Autodesk Inventor part; units mm, degrees
ref_plane "YZ Plane" through (0, 0, 0) normal (1, 0, 0) x (0, 1, 0)
ref_plane "XZ Plane" through (0, 0, 0) normal (0, 1, 0) x (-1, 0, 0)
ref_plane "XY Plane" through (0, 0, 0) normal (0, 0, 1) x (1, 0, 0)
sketch "Эскиз1" plane through (0, 0, 0) normal (0, 0, 1) x (1, 0, 0)
  circle A0 centre (0, 0) radius 40
  line L0 (-40, 0) -> (-13.6038, 219.402)
  line L1 (-13.6038, 219.402) -> (13.6038, 219.402)
  line L2 (13.6038, 219.402) -> (40, 0)
  line L3 (0, 0) -> (0, 40) construction
  line L4 (0, 0) -> (40, 0) construction
  point P0 (0, 219.402)
  dimension "d0" = 80
extrude "Выдавливание1" add sketch "Эскиз1" along normal blind 3 contours L0 A0 L2 | L0 L1 L2 A0
sketch "Эскиз2" plane through (0, 0, 3) normal (0, 0, 1) x (1, 0, 0)
  arc A0 (3, 2.25) -> (-3, 2.25) centre (0, 0) ccw construction
  line L0 (-1.9929, 14.1684) -> (-3, 2.25) construction
  arc A1 (1.9929, 14.1684) -> (-1.9929, 14.1684) centre (0, 14) ccw construction
  line L1 (3, 2.25) -> (1.9929, 14.1684) construction
  circle A2 centre (0, 13) radius 0.5 construction
  circle A3 centre (0, 11) radius 0.5 construction
  circle A4 centre (0, 9) radius 0.5 construction
  circle A5 centre (0, 7) radius 0.5 construction
  circle A6 centre (0, 5) radius 0.5 construction
  circle A7 centre (0, 15) radius 0.5 construction
  arc A8 (-1.9929, -14.1684) -> (1.9929, -14.1684) centre (0, -14) ccw construction
  line L2 (-3, -2.25) -> (-1.9929, -14.1684) construction
  arc A9 (-3, -2.25) -> (3, -2.25) centre (0, 0) ccw construction
  line L3 (1.9929, -14.1684) -> (3, -2.25) construction
  circle A10 centre (0, -5) radius 0.5 construction
  circle A11 centre (0, -7) radius 0.5 construction
  circle A12 centre (0, -9) radius 0.5 construction
  circle A13 centre (0, -11) radius 0.5 construction
  circle A14 centre (0, -13) radius 0.5 construction
  circle A15 centre (0, -15) radius 0.5 construction
  circle A16 centre (0, 0) radius 2.3
  circle A17 centre (0, 9) radius 1
  circle A18 centre (0, -9) radius 1
  point P0 (0, 0)
  dimension "d3" = 2
  dimension "d4" = 2
extrude "Выдавливание2" cut sketch "Эскиз2" against normal blind 10
properties part number "ухо"
Check sheet for the modelled part. Datum: model origin and axes. Units: mm. Give positions to 0.01 mm unless a question says otherwise; leave off trailing zeros. Order: outer loops, then holes, each group sorted by start corner. A loop starts at its lowest first (then second) coordinate and runs counter-clockwise, first axis right, second up. Notation, with made-up numbers: M 56,32 L 97,32 A22 cw 97,40 Z; hole C -9.75,17.5 d11. An arc over 180 degrees is marked long. Answer in a Markdown table with one row per item.
1) Cross-section at A-A, the plane z = 0.8. Enter the section's corners in (x, y).
Filled sheet:
| item | result |
|---|---|
| outline | M -40,0 A40 ccw 40,0 L 13.6,219.4 L -13.6,219.4 Z; hole C 0,0 d4.6; hole C 0,-9 d2; hole C 0,9 d2 |
2) Release check for a two-part mould opening along X. For faces 1 (the cylindrical face through (-1.825, -1.4, 1.521)), 2 (the flat face through (-26.987, 108.165, 1.479)), 3 (the flat face through (-1, 63, 0)) record: +X half, -X half, draft (parallel to the pull), parting line (faces both ways), or undercut.
Filled sheet:
| item | result |
|---|---|
| face 1 | undercut |
| face 2 | -X half |
| face 3 | draft |
3) Cross-section at B-B, the plane x = -20.5. Enter the section's corners in (y, z), plus the area to 3 significant figures.
Filled sheet:
| item | result |
|---|---|
| outline | M -34.35,0 L 162.08,0 L 162.08,3 L -34.35,3 Z |
| area | 589 mm2 |
4) Cross-section at C-C, the plane y = 165. Enter the section's corners in (x, z), plus the area to 3 significant figures.
Filled sheet:
| item | result |
|---|---|
| outline | M -20.15,0 L 20.15,0 L 20.15,3 L -20.15,3 Z |
| area | 121 mm2 |
5) Thickness scan on L1, parallel to Y at x = 0, z = 2.3; L2, parallel to X at y = 148.5, z = 2.75; L3, parallel to X at y = 48, z = 0.4. Record the ranges inside material, lowest first. Write a range as [from, to].
Filled sheet:
| item | result |
|---|---|
| L1 | y = [-40, -10], [-8, -2.3], [2.3, 8], [10, 219.4] |
| L2 | x = [-22.13, 22.13] |
| L3 | x = [-34.23, 34.23] |
6) Gauge pin test, flat ends, axial feed: P1, Ø2.5, axis at x = 0, y = 9, coming from the +Z side; P2, Ø4, axis at x = 0, y = 0, coming from the +Z side; P3, Ø1.5, axis at x = -1.5, z = 0.5, coming from the -Y side. Record the tip position at first contact, or that the pin passes through.
Filled sheet:
| item | result |
|---|---|
| P1 | stops at z = 3 |
| P2 | passes through |
| P3 | stops at y = -39.99 |
